Build history of the part. All positions in model axes, mm. A direction names the side the tool comes from. Round coordinates to 2 decimals unless told otherwise and drop trailing zeros. Order: outer loops, then holes, each group sorted by start corner. A loop starts at its lowest first (then second) coordinate and runs counter-clockwise, first axis right, second up. Notation, with made-up numbers: (78.5, 21.25) -> (131.5, 21.25) arc R12 ccw to (131.5, 36.25) -> close; hole circle Ø9 at (-34, 84.5). An arc over 180 degrees is marked (long way). Answer as a JSON object with one key per item and string values.
from build123d import *

# Parameters (mm, degrees)
SKETCH1_W            = 141.6
SKETCH1_H            = 41.9
BOSS_EXTRUDE1_DEPTH  = 28
SKETCH2_W            = 11
SKETCH2_H            = 0.5
BOSS_EXTRUDE2_DEPTH  = 9.05
FILLET1_R            = 2
SKETCH3_W            = 4
SKETCH3_H            = 4.2
CUT_EXTRUDE1_DEPTH   = 9.05
FILLET1_OF_MIRROR1_R = 2
MIRROR2_DEPTH        = 0.5


# Read off the part's stored shape, not the designer's step: Mirror2
with BuildPart() as part:
    # Sketch1 → Boss-Extrude1 (new body)
    with BuildSketch(Plane(origin=(0, 0, 0), x_dir=(1, 0, 0), z_dir=(0, 1, 0))):
        Rectangle(SKETCH1_W, SKETCH1_H)
    extrude(amount=BOSS_EXTRUDE1_DEPTH)

    # Sketch2 → Boss-Extrude2 (add)
    with BuildSketch(Plane.XY.offset(20.95)):
        with Locations((-65.3, 0.25)):
            Rectangle(SKETCH2_W, SKETCH2_H)
    boss_extrude2 = extrude(amount=BOSS_EXTRUDE2_DEPTH)

    # Fillet1
    fillet1_edges = [part.edges().sort_by_distance(p)[0] for p in [
        (-59.8, 0.25, 30),
        (-70.8, 0.25, 30),
    ]]
    fillet(fillet1_edges, radius=FILLET1_R)

    # Sketch3 → Cut-Extrude1 (cut)
    with BuildSketch(Plane(origin=(0, 0.5, 0), x_dir=(1, 0, 0), z_dir=(0, 1, 0))):
        with BuildLine():
            ThreePointArc((-67.3, -25.8), (-65.3, -23.8), (-63.3, -25.8))
            Line((-63.3, -25.8), (-67.3, -25.8))
        make_face()
        with Locations((-65.3, -27.9)):
            Rectangle(SKETCH3_W, SKETCH3_H)
    cut_extrude1 = extrude(amount=-CUT_EXTRUDE1_DEPTH, mode=Mode.SUBTRACT)

    # Mirror1: Boss-Extrude2, Cut-Extrude1 across plane
    add(boss_extrude2.mirror(Plane(origin=(0, 0, 0), x_dir=(0, 0, 1), z_dir=(1, 0, 0))))
    add(cut_extrude1.mirror(Plane(origin=(0, 0, 0), x_dir=(0, 0, 1), z_dir=(1, 0, 0))), mode=Mode.SUBTRACT)

    # Fillet1 of Mirror1
    fillet1_of_mirror1_edges = [part.edges().sort_by_distance(p)[0] for p in [
        (59.8, 0.25, 30),
        (70.8, 0.25, 30),
    ]]
    fillet(fillet1_of_mirror1_edges, radius=FILLET1_OF_MIRROR1_R)

    # Mirror2 outline → Mirror2 (add)
    with BuildSketch(Plane(origin=(0, 0, 0), x_dir=(1, 0, 0), z_dir=(0, 1, 0))):
        with BuildLine():
            Line((59.8, 28), (59.8, 20.95))
            Line((59.8, 20.95), (70.8, 20.95))
            Line((70.8, 20.95), (70.8, 28))
            ThreePointArc((70.8, 28), (70.214213562, 29.414213562), (68.8, 30))
            Line((68.8, 30), (67.3, 30))
            Line((67.3, 30), (67.3, 25.8))
            ThreePointArc((67.3, 25.8), (65.3, 23.8), (63.3, 25.8))
            Line((63.3, 25.8), (63.3, 30))
            Line((63.3, 30), (61.8, 30))
            ThreePointArc((61.8, 30), (60.385786438, 29.414213562), (59.8, 28))
        make_face()
        with BuildLine():
            Line((-67.3, 30), (-68.8, 30))
            ThreePointArc((-68.8, 30), (-70.214213562, 29.414213562), (-70.8, 28))
            Line((-70.8, 28), (-70.8, 20.95))
            Line((-70.8, 20.95), (-59.8, 20.95))
            Line((-59.8, 20.95), (-59.8, 28))
            ThreePointArc((-59.8, 28), (-60.385786438, 29.414213562), (-61.8, 30))
            Line((-61.8, 30), (-63.3, 30))
            Line((-63.3, 30), (-63.3, 25.8))
            ThreePointArc((-63.3, 25.8), (-65.3, 23.8), (-67.3, 25.8))
            Line((-67.3, 25.8), (-67.3, 30))
        make_face()
    extrude(amount=MIRROR2_DEPTH)


solid = part.part
1) Probe L1, parallel to Z at x = -21.5, y = 9.25. List the from-to ranges inside material, lowest first. Write a range as from..to.
Checked values:
{"L1": "z = -20.95..20.95"}
2) Cut at A-A, the plane x = -65.3. Give the cut face in (y, z), plus the area to 3 significant figures.
Checked values:
{"outline": "(0, -23.8) -> (0.5, -23.8) -> (0.5, -20.95) -> (28, -20.95) -> (28, 20.95) -> (0.5, 20.95) -> (0.5, 23.8) -> (0, 23.8) -> close", "area": "1,180 mm²"}
3) Cut at B-B, the plane y = 9. Give the cut face in (x, z).
Checked values:
{"outline": "(-70.8, -20.95) -> (70.8, -20.95) -> (70.8, 20.95) -> (-70.8, 20.95) -> close"}
4) Which spindle directions (+Z, -Z, +X, -X, +Y, -Y) get a long thin tool onto all of the face, cutting with end or side? Do faces 1 (the face through (65, 0.5, 23)), 2 (the face through (65.2, 0.5, -23.5)), 3 (the face through (-1, 0, 0)). Say none if no direction does.
Checked values:
{"face 1": "+Z, +X, -X, +Y", "face 2": "-Z, +X, -X, +Y", "face 3": "+Z, -Z, +X, -X, -Y"}
5) Flat gauge pins, fed straight in: pin 1 Ø2.5 at (x, z) = (-63.5, 23.5) entering from +Y; pin 2 Ø5 at (x, z) = (31, -17) entering from -Y; pin 3 Ø2 at (x, z) = (51.5, 23) entering from -Y; pin 4 Ø5 at (x, y) = (-39, 12) entering from -Z. Where does each tip first touch, or does it go through?
Checked values:
{"pin 1": "stops at y = 0.5", "pin 2": "stops at y = 0", "pin 3": "passes through", "pin 4": "stops at z = -20.95"}
6) Cut at C-C, the plane x = 12. Give the cut face in (y, z).
Checked values:
{"outline": "(0, -20.95) -> (28, -20.95) -> (28, 20.95) -> (0, 20.95) -> close"}
